Design review of the part built by this model. Coordinates are the model's own, in mm. A direction names the side the tool comes from. Coordinates: 2 decimals unless noted, no trailing zeros. Loops run counter-clockwise (first coordinate to the right, second up) from the corner with the lowest first, then second, coordinate; pieces in that order, holes last. Notation, with made-up numbers: (6, -30.75) -> (45, -30.75) arc R17 cw to (45, -20.75) -> close; hole circle Ø5 at (39.25, 69). An arc over 180 degrees is marked (long way). One line per item, written item: value. Start each with the question number.
1. Add section C-C on x = 39.5. Write out the cut boundary in (y, z), plus the area to 3 significant figures.
2. Add section D-D on x = 74.5. Write out the cut boundary in (y, z), plus the area to 3 significant figures.
3. Add section A-A on y = 10.5. Write out the cut boundary in (x, z), plus the area to 3 significant figures.
4. Machinability: for faces 5 (the cylindrical face through (84.14, 21.9, 5.04)), 6 (the flat face through (4, 47, 3)), 7 (the cylindrical face through (33, 2, 4)), which of the approach directions +Z, -Z, +X, -X, +Y, -Y give a long, thin tool a straight path to every point of the face, cutting with its end or side? Answer none if there is none.
5. Add section B-B on z = 6. Write out the cut boundary in (x, y), plus the area to 3 significant figures.
6. For probe 1 along Y at (x, z) = (5, 7); probe 2 along X at (y, z) = (4, 8.25); probe 3 along Z at (x, y) = (63, 34), list the stretches that pass through material, from the lowest coordinate up.
7. Insertion check: pin 1 (0.5 mm diameter, centred on y = 38.5, z = 2.5, fed in from +X); pin 2 (0.8 mm diameter, centred on y = 8, z = 8.5, fed in from -X); pin 3 (25 mm diameter, centred on x = 27.5, y = 11, fed in from +Z). Each pin has a flat end and moves straight along its axis. Give the tip position at first contact, or say it passes through.
8. Draft analysis for pull direction X (two halves, no side actions). For faces 1 (the cylindrical face through (84.14, 0.9, 3.94)), 2 (the flat face through (4, 12, 9)), 3 (the flat face through (43, 12, 8)), 4 (the cylindrical face through (0.9, 21.94, 5.04)), state which applies: pulls with the +X half, pulls with the -X half, needs draft (parallel to the pull), parting line crosses it, or undercut.
```python
from build123d import *

# Parameters (mm, degrees)
BOSS_EXTRUDE1_DEPTH = 8
CUT_EXTRUDE1_DEPTH  = 6
SKETCH3_W           = 2.01
SKETCH3_H           = 16.8
BOSS_EXTRUDE2_DEPTH = 1
SKETCH4_W           = 2.01
SKETCH4_H           = 40.8
BOSS_EXTRUDE3_DEPTH = 1


with BuildPart() as part:
    # Sketch1 → Boss-Extrude1 (new body)
    with BuildSketch(Plane.XY):
        with BuildLine():
            Line((3, 70), (82, 70))
            ThreePointArc((82, 70), (84.121320344, 69.121320344), (85, 67))
            Line((85, 67), (85, 3))
            ThreePointArc((85, 3), (84.121320344, 0.878679656), (82, 0))
            Line((82, 0), (52.7, 0))
            ThreePointArc((52.7, 0), (51.7627417, 2.2627417), (49.5, 3.2))
            Line((49.5, 3.2), (35.5, 3.2))
            ThreePointArc((35.5, 3.2), (33.2372583, 2.2627417), (32.3, 0))
            Line((32.3, 0), (3, 0))
            ThreePointArc((3, 0), (0.878679656, 0.878679656), (0, 3))
            Line((0, 3), (0, 67))
            ThreePointArc((0, 67), (0.878679656, 69.121320344), (3, 70))
        make_face()
    extrude(amount=BOSS_EXTRUDE1_DEPTH)

    # Sketch2 → Cut-Extrude1 (cut)
    with BuildSketch(Plane.XY.offset(8)):
        with BuildLine():
            Line((3, 70), (82, 70))
            ThreePointArc((82, 70), (84.121320344, 69.121320344), (85, 67))
            Line((85, 67), (85, 19.8))
            ThreePointArc((85, 19.8), (84.121320344, 21.921320344), (82, 22.8))
            Line((82, 22.8), (3, 22.8))
            ThreePointArc((3, 22.8), (0.878679656, 21.921320344), (0, 19.8))
            Line((0, 19.8), (0, 67))
            ThreePointArc((0, 67), (0.878679656, 69.121320344), (3, 70))
        make_face()
    extrude(amount=-CUT_EXTRUDE1_DEPTH, mode=Mode.SUBTRACT)

    # Sketch3 → Boss-Extrude2 (add)
    with BuildSketch(Plane.XY.offset(8)):
        with Locations((4.105, 11.5)):
            Rectangle(SKETCH3_W, SKETCH3_H)
        with Locations((80.895, 11.5)):
            Rectangle(SKETCH3_W, SKETCH3_H)
    extrude(amount=BOSS_EXTRUDE2_DEPTH)

    # Sketch4 → Boss-Extrude3 (add)
    with BuildSketch(Plane.XY.offset(2)):
        with Locations((4.105, 46.5)):
            Rectangle(SKETCH4_W, SKETCH4_H)
        with Locations((80.895, 46.5)):
            Rectangle(SKETCH4_W, SKETCH4_H)
    extrude(amount=BOSS_EXTRUDE3_DEPTH)


solid = part.part
```
Worked answers:
1. outline: (3.2, 0) -> (70, 0) -> (70, 2) -> (22.8, 2) -> (22.8, 8) -> (3.2, 8) -> close
1. area: 251 mm²
2. outline: (0, 0) -> (70, 0) -> (70, 2) -> (22.8, 2) -> (22.8, 8) -> (0, 8) -> close
2. area: 277 mm²
3. outline: (0, 0) -> (85, 0) -> (85, 8) -> (81.9, 8) -> (81.9, 9) -> (79.89, 9) -> (79.89, 8) -> (5.11, 8) -> (5.11, 9) -> (3.1, 9) -> (3.1, 8) -> (0, 8) -> close
3. area: 684 mm²
4. face 5: +Z, +X, +Y
4. face 6: +Z, +X, -X, +Y
4. face 7: +Z, -Z, -Y
5. outline: (0, 3) arc R3 ccw to (3, 0) -> (32.3, 0) arc R3.2 cw to (35.5, 3.2) -> (49.5, 3.2) arc R3.2 cw to (52.7, 0) -> (82, 0) arc R3 ccw to (85, 3) -> (85, 19.8) arc R3 ccw to (82, 22.8) -> (3, 22.8) arc R3 ccw to (0, 19.8) -> close
5. area: 1,870 mm²
6. probe 1: y = 0 to 22.8
6. probe 2: x = 3.1 to 5.11, 79.89 to 81.9
6. probe 3: z = 0 to 2
7. pin 1: stops at x = 81.9
7. pin 2: stops at x = 3.1
7. pin 3: stops at z = 8
8. face 1: pulls with the +X half
8. face 2: needs draft
8. face 3: undercut
8. face 4: pulls with the -X half
